Geometry: final body of the model. Coordinates: model frame, mm. A direction names the side the tool comes from. Give positions to 0.01 mm unless a question says otherwise; leave off trailing zeros. Loops run counter-clockwise (first coordinate to the right, second up) from the corner with the lowest first, then second, coordinate; pieces in that order, holes last.
1. Material intervals for line 1 along Y through (x, z) = (3.5, 0); line 2 along X through (y, z) = (18, -1.75); line 3 along Z through (x, y) = (0, 13), sorted ascending.
2. First-contact query: P1, Ø2, axis at y = 10.5, z = -2.5, coming from the -X side. Flat tip, straight axial feed; report the tip coordinate or a pass-through.
3. Section A-A, the plane x = 0. Output: boundary loops of the cut face in (y, z), then the cut area to 3 significant figures.
4. Section C-C, the plane y = 14. Output: boundary loops of the cut face in (x, z), then the cut area to 3 significant figures.
5. Section B-B, the plane z = 0. Output: boundary loops of the cut face in (x, y), then the cut area to 3 significant figures.
6. Access query for faces 1 (the face through (-2.038, 24.262, -2.658)), 2 (the face through (-2.038, 2.958, -2.658)), 3 (the face through (0.165, 6.74, 3.746)). Directions: +Z, -Z, +X, -X, +Y, -Y. A direction counts if a zero-diameter tool reaches every point of the face in a straight line with its end or side. Return the directions, or none.
from build123d import *

# Parameters (mm, degrees)
SKETCH1_R           = 3.35
BOSS_EXTRUDE1_DEPTH = 42
SKETCH4_R           = 3.75
BOSS_EXTRUDE3_DEPTH = 1.5
FILLET1_R           = 0.5


with BuildPart() as part:
    # Sketch1 → Boss-Extrude1 (new body)
    with BuildSketch(Plane(origin=(0, 0, 0), x_dir=(1, 0, 0), z_dir=(0, 1, 0))):
        with Locations(Location((0, 0, 0), (0, 0, 270))):  # turned: the seam where the file's is
            Circle(SKETCH1_R)
    extrude(amount=BOSS_EXTRUDE1_DEPTH)

    # Sketch4 → Boss-Extrude3 (add)
    with BuildSketch(Plane(origin=(0, 6, 0), x_dir=(-1, 0, 0), z_dir=(0, -1, 0))):
        with Locations(Location((0, 0, 0), (0, 0, 90))):  # turned: the seam where the file's is
            Circle(SKETCH4_R)
    extrude(amount=-BOSS_EXTRUDE3_DEPTH)

    # Fillet1
    fillet1_edges = [part.edges().sort_by_distance(p)[0] for p in [
        (0, 42, -3.35),
    ]]
    fillet(fillet1_edges, radius=FILLET1_R)


solid = part.part
Answers below:
1. line 1: y = 6 to 7.5
1. line 2: x = -2.86 to 2.86
1. line 3: z = -3.35 to 3.35
2. P1: stops at x = -3
3. outline: (0, -3.35) - (6, -3.35) - (6, -3.75) - (7.5, -3.75) - (7.5, -3.35) - (41.5, -3.35) arc R0.5 ccw to (42, -2.85) - (42, 2.85) arc R0.5 ccw to (41.5, 3.35) - (7.5, 3.35) - (7.5, 3.75) - (6, 3.75) - (6, 3.35) - (0, 3.35) - close
3. area: 282 mm2
4. outline: circle Ø6.7 at (0, 0)
4. area: 35.3 mm2
5. outline: (-3.75, 6) - (-3.35, 6) - (-3.35, 0) - (3.35, 0) - (3.35, 6) - (3.75, 6) - (3.75, 7.5) - (3.35, 7.5) - (3.35, 41.5) arc R0.5 ccw to (2.85, 42) - (-2.85, 42) arc R0.5 ccw to (-3.35, 41.5) - (-3.35, 7.5) - (-3.75, 7.5) - close
5. area: 282 mm2
6. face 1: +Y
6. face 2: -Y
6. face 3: +Y, -Y
